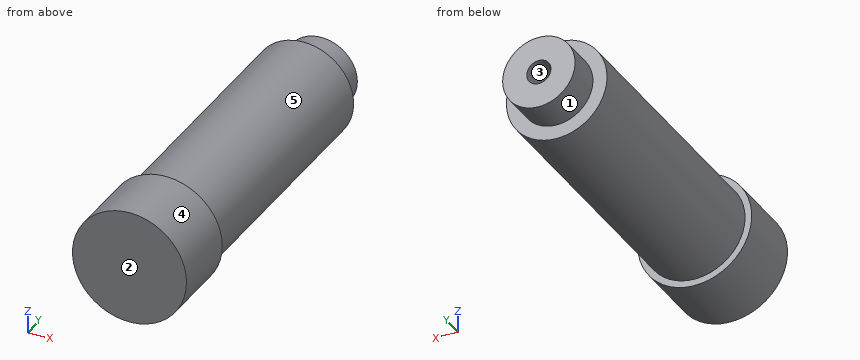
Autodesk Inventor part; units mm, degrees
ref_plane "YZ Plane" through (0, 0, 0) normal (1, 0, 0) x (0, 1, 0)
ref_plane "XZ Plane" through (0, 0, 0) normal (0, 1, 0) x (-1, 0, 0)
ref_plane "XY Plane" through (0, 0, 0) normal (0, 0, 1) x (1, 0, 0)
sketch "Boceto1" plane through (0, 0, 0) normal (0, 1, 0) x (-1, 0, 0)
  circle A0 centre (0, 0) radius 6.05
  dimension "d0" = 12.1
extrude "Extrusión1" add sketch "Boceto1" against normal blind 32.4
sketch "Boceto2" plane through (0, 0, 0) normal (0, 1, 0) x (1, 0, 0)
  circle A0 centre (0, 0) radius 4.35
  dimension "d3" = 8.7
extrude "Extrusión2" add sketch "Boceto2" along normal blind 4.2
thread "Rosca1"
sketch "Boceto3" plane through (0, -32.4, 0) normal (0, -1, 0) x (1, 0, 0)
  circle A0 centre (0, 0) radius 6.9
  dimension "d8" = 13.8
sketch "Boceto4" plane through (0, -32.4, 0) normal (0, -1, 0) x (1, 0, 0)
  circle A0 centre (0, 0) radius 5.95
  dimension "d9" = 11.9
extrude "Extrusión3" cut sketch "Boceto4" against normal blind 28.7
sketch "Boceto5" plane through (0, -32.4, 0) normal (0, -1, 0) x (1, 0, 0)
  point P0 (0, 0)
extrude "Extrusión4" add sketch "Boceto3" along normal blind 8.4
sketch "Boceto6" plane through (0, 4.2, 0) normal (0, 1, 0) x (1, 0, 0)
  circle A0 centre (0, 0) radius 1.45
  dimension "d14" = 2.9
extrude "Extrusión5" cut sketch "Boceto6" against normal blind 20
sketch "Boceto7" plane through (0, -40.8, 0) normal (0, -1, 0) x (1, 0, 0)
  circle A0 centre (0, 0) radius 6.85
  circle A1 centre (0, 0) radius 6.9
  dimension "d17" = 13.7
  dimension "d18" = 13.8
extrude "Extrusión6" cut sketch "Boceto7" against normal blind 20
properties part number "Piston(Deposito_deAceite)" material "Plástico ABS"
The model under review builds one solid part; all positions refer to its coordinate system, in mm. Face numbers are marked on the shaded views. A direction names the side the tool comes from. Round coordinates to 2 decimals unless told otherwise and drop trailing zeros. Write each loop counter-clockwise with the first axis right and the second up, starting at its lowest first coordinate (ties: lowest second). Pieces come first, ordered by that corner, then holes.
(1) Mouldability with a two-part tool opening along Z and no side actions: class the marked faces 1, 2 and 3 as +Z half, -Z half, draft (parallel to the pull), parting line (faces both ways), or undercut.
(2) Machinability: for the marked faces 4 and 5, which of the approach directions +Z, -Z, +X, -X, +Y, -Y give a long, thin tool a straight path to every point of the face, cutting with its end or side? Answer none if there is none.
(3) We need section B-B on z = 0. Give the boundary of the cut face in (x, y).
(4) We need section C-C on y = -26. Give the boundary of the cut face in (x, z).
(5) We need section A-A on x = 0. Give the boundary of the cut face in (y, z).
(6) Wall thickness on L1, parallel to Y at x = 1.25, z = 1; L2, parallel to Y at x = 2, z = 5.5; L3, parallel to Z at x = 0, y = 2: over which ranges is each line inside the solid? List them lowest first.
(7) Insertion check: pin 1 (2 mm diameter, centred on y = -22, z = 5, fed in from +X); pin 2 (2 mm diameter, centred on y = -34.5, z = 4.5, fed in from -X); pin 3 (3 mm diameter, centred on y = -13, z = 4, fed in from -X). Each pin has a flat end and moves straight along its axis. Give the tip position at first contact, or say it passes through.
Findings below:
1. face 1: parting line
1. face 2: draft
1. face 3: undercut
2. face 4: +Y, -Y
2. face 5: +Y
3. outline: (-6.85, -40.8) - (6.85, -40.8) - (6.85, -32.4) - (6.05, -32.4) - (6.05, 0) - (4.35, 0) - (4.35, 4.2) - (1.45, 4.2) - (1.45, -3.7) - (5.95, -3.7) - (5.95, -32.4) - (-5.95, -32.4) - (-5.95, -3.7) - (-1.45, -3.7) - (-1.45, 4.2) - (-4.35, 4.2) - (-4.35, 0) - (-6.05, 0) - (-6.05, -32.4) - (-6.85, -32.4) - close
4. outline: circle Ø12.1 at (0, 0); hole circle Ø11.9 at (0, 0)
5. outline: (-40.8, -6.85) - (-32.4, -6.85) - (-32.4, -6.05) - (0, -6.05) - (0, -4.35) - (4.2, -4.35) - (4.2, -1.45) - (-3.7, -1.45) - (-3.7, -5.95) - (-32.4, -5.95) - (-32.4, 5.95) - (-3.7, 5.95) - (-3.7, 1.45) - (4.2, 1.45) - (4.2, 4.35) - (0, 4.35) - (0, 6.05) - (-32.4, 6.05) - (-32.4, 6.85) - (-40.8, 6.85) - close
6. L1: y = -40.8 to -32.4, -3.7 to 4.2
6. L2: y = -40.8 to -32.4, -3.7 to 0
6. L3: z = -4.35 to -1.45, 1.45 to 4.35
7. pin 1: stops at x = 4.54
7. pin 2: stops at x = -5.89
7. pin 3: stops at x = -5.51
